```python
from build123d import *


with BuildPart() as part:
    # Çizim1 → Döndür1 (revolve)
    with BuildSketch(Plane.XY):
        with BuildLine():
            Line((38, 0), (38, 12))
            Line((38, 12), (28, 12))
            Line((28, 12), (28, 89))
            ThreePointArc((28, 89), (25.656854249, 94.656854249), (20, 97))
            Line((20, 97), (18, 97))
            Line((18, 97), (18, 100))
            ThreePointArc((18, 100), (17.414213562, 101.414213562), (16, 102))
            Line((16, 102), (11.5, 102))
            Line((11.5, 102), (11.5, 87))
            Line((11.5, 87), (20, 87))
            ThreePointArc((20, 87), (21.414213562, 86.414213562), (22, 85))
            Line((22, 85), (22, 43))
            ThreePointArc((22, 43), (21.414213562, 41.585786438), (20, 41))
            Line((20, 41), (6, 41))
            Line((6, 41), (6, 31))
            Line((6, 31), (20, 31))
            ThreePointArc((20, 31), (21.414213562, 30.414213562), (22, 29))
            Line((22, 29), (22, 3))
            Line((22, 3), (35, 3))
            Line((35, 3), (35, 0))
            Line((35, 0), (38, 0))
        make_face()
    revolve(axis=Axis((0, 0, 0), (0, 1, 0)))


solid = part.part
```
For this review, take the finished solid that the model builds, in its own axes (mm). A direction names the side the tool comes from. Round coordinates to 2 decimals unless told otherwise and drop trailing zeros. Write each loop counter-clockwise with the first axis right and the second up, starting at its lowest first coordinate (ties: lowest second). Pieces come first, ordered by that corner, then holes. Notation, with made-up numbers: (63, 8) - (102, 8) arc R20 cw to (102, 15) - close; hole circle Ø7 at (63, -1). An arc over 180 degrees is marked (long way). Answer as a JSON object with one key per item and string values.
1. We need section A-A on x = -31.5. Give the boundary of the cut face in (y, z).
Response values:
{"outline": "(0, -21.25) - (12, -21.25) - (12, 21.25) - (0, 21.25) - (0, 15.26) - (3, 15.26) - (3, -15.26) - (0, -15.26) - close"}
2. Draft analysis for pull direction Y (two halves, no side actions). For faces 4 (the face through (4, 41, -5)), 5 (the face through (25.865, 51.039, 10.724)), 6 (the face through (-11, 102, -4)), state which applies: +Y half, -Y half, draft (parallel to the pull), parting line (faces both ways), or undercut.
Response values:
{"face 4": "undercut", "face 5": "draft", "face 6": "+Y half"}
3. We need section C-C on z = -30. Give the boundary of the cut face in (x, y), then the cut area to 3 significant figures.
Response values:
{"outline": "(-23.32, 0) - (-18.03, 0) - (-18.03, 3) - (18.03, 3) - (18.03, 0) - (23.32, 0) - (23.32, 12) - (-23.32, 12) - close", "area": "452 mm2"}
4. Tool access review of faces 1 (the face through (-9, 87, 9)), 2 (the face through (0, 3, 23)), 3 (the face through (-3, 12, 28)): name each direction out of +Z, -Z, +X, -X, +Y, -Y from which nothing blocks a thin tool from reaching the whole face with its end or side.
Response values:
{"face 1": "none", "face 2": "-Y", "face 3": "+Y"}
5. We need section B-B on y = 14. Give the boundary of the cut face in (x, z).
Response values:
{"outline": "circle Ø56 at (0, 0); hole circle Ø44 at (0, 0)"}
6. For pin 1 Ø1.5 at (y, z) = (28, -24.5) entering from -X; pin 2 Ø2 at (y, z) = (74, -19) entering from +X; pin 3 Ø14 at (x, z) = (0, 0) entering from -Y, all flat-tipped, find the tip position at first contact; note any pin that passes through.
Response values:
{"pin 1": "stops at x = -14.83", "pin 2": "stops at x = 21.45", "pin 3": "stops at y = 31"}
7. To check wall thickness, follow line 1 along Z through (x, y) = (0, 37); line 2 along X through (y, z) = (13, 0). State the ranges of each line that lie inside material, in increasing order.
Response values:
{"line 1": "z = -28 to -6, 6 to 28", "line 2": "x = -28 to -22, 22 to 28"}
